Geometry: final body of the model. Coordinates: model frame, mm. A direction names the side the tool comes from. Give positions to 0.01 mm unless a question says otherwise; leave off trailing zeros. Write each loop counter-clockwise with the first axis right and the second up, starting at its lowest first coordinate (ties: lowest second). Pieces come first, ordered by that corner, then holes. Notation, with made-up numbers: M 81,36.5 L 137,36.5 A32 cw 137,62.5 Z; hole C -8,-39 d2. An arc over 180 degrees is marked long. Use a Markdown table: item, result. Add a question column.
1) Line query: line 1 (Y direction, x = -5, z = 27); line 2 (X direction, y = -3.5, z = 4.5); line 3 (X direction, y = -14, z = 16). Output: solid intervals per line, ascending.
2) Section B-B on z = 8. Return the cut outline in (x, y), then the cut area to 3 significant figures.
3) Section D-D on y = 15. Return the cut outline in (x, z).
4) Set-up query: faces 4 (the flat face through (-4, -13.5, 19)), 5 (the flat face through (-1, 0, 23)), 6 (the flat face through (-0.5, 3.15, 34.9)), 7 (the flat face through (-0.5, 3.15, 12.6)). Return all of +Z, -Z, +X, -X, +Y, -Y with unobstructed straight access to the full face (end or side cutting, diameter ignored); none if empty.
5) Pin query (flat end, axial travel): pin 1 (2.5 mm diameter, centred on x = -3, z = 19.5, fed in from -Y); pin 2 (3 mm diameter, centred on y = 16.5, z = 18.5, fed in from +X); pin 3 (2 mm diameter, centred on y = 2, z = 29.5, fed in from -X); pin 4 (3 mm diameter, centred on y = -0.5, z = 6.5, fed in from +X). Return the tip coordinate at first contact, or that it passes through.
6) Section A-A on x = -3.25. Return the cut outline in (y, z), then the cut area to 3 significant figures.
7) Draft query along Z for faces 1 (the cylindrical face through (-0.5, -0.1, 21.5)), 2 (the flat face through (-0.7, 0.1, 0)), 3 (the flat face through (-4, 13.5, 19)). Return one class per face: +Z half, -Z half, draft (parallel to the pull), parting line (faces both ways), or undercut.
8) Section C-C on z = 27.5. Return the cut outline in (x, y), then the cut area to 3 significant figures.
```python
from build123d import *

# Parameters (mm, degrees)
EXTRUDE_THIN1_DEPTH = 50.8
CUT_EXTRUDE1_START  = -8.5
CUT_EXTRUDE1_DEPTH  = 9.5
LPATTERN1_COUNT     = 2
LPATTERN1_PITCH     = 25
FILLET1_R           = 0.25
FILLET2_R           = 1.25
SKETCH5_W           = 12.8
SKETCH5_H           = 35
CUT_EXTRUDE2_DEPTH  = 8.5


with BuildPart() as part:
    # Sketch3 → Extrude-Thin1 (new body)
    with BuildSketch(Plane.XY):
        Polygon((-6.5, 17.5), (-6.5, 13.5), (0, 13.5), (0, -13.5), (-6.5, -13.5), (-6.5, -17.5), (-7.5, -17.5), (-7.5, -12.5), (-1, -12.5), (-1, 12.5), (-7.5, 12.5), (-7.5, 17.5), align=None)
    extrude(amount=EXTRUDE_THIN1_DEPTH)

    # Sketch4 → Cut-Extrude1 (cut)
    with BuildSketch(Plane(origin=(0, 0, 0), x_dir=(0, 0, -1), z_dir=(1, 0, 0)).offset(CUT_EXTRUDE1_START)):
        with BuildLine():
            Line((-6.65, -3.15), (-18.35, -3.15))
            ThreePointArc((-18.35, -3.15), (-21.5, 0), (-18.35, 3.15))
            Line((-18.35, 3.15), (-6.65, 3.15))
            ThreePointArc((-6.65, 3.15), (-3.5, 0), (-6.65, -3.15))
        make_face()
    cut_extrude1 = extrude(amount=CUT_EXTRUDE1_DEPTH, mode=Mode.SUBTRACT)

    # LPattern1: Cut-Extrude1 ×2
    with Locations(*[(0, 0, i * LPATTERN1_PITCH) for i in range(1, LPATTERN1_COUNT)]):
        add(cut_extrude1, mode=Mode.SUBTRACT)

    # Fillet1
    fillet1_edges = [part.edges().sort_by_distance(p)[0] for p in [
        (-6.5, 13.5, 25.4),
        (-6.5, -13.5, 25.4),
        (-1, -12.5, 25.4),
        (-1, 12.5, 25.4),
    ]]
    fillet(fillet1_edges, radius=FILLET1_R)

    # Fillet2
    fillet2_edges = [part.edges().sort_by_distance(p)[0] for p in [
        (0, 13.5, 25.4),
        (0, -13.5, 25.4),
        (-7.5, -12.5, 25.4),
        (-7.5, 12.5, 25.4),
    ]]
    fillet(fillet2_edges, radius=FILLET2_R)

    # Sketch5 → Cut-Extrude2 (cut, through all)
    with BuildSketch(Plane.ZY.offset(7.5)):
        with Locations((44.4, 0)):
            Rectangle(SKETCH5_W, SKETCH5_H)
    extrude(amount=-CUT_EXTRUDE2_DEPTH, mode=Mode.SUBTRACT)


solid = part.part
```
Found:
| question | item | result |
|---|---|---|
| 1 | line 1 | -13.5 to -12.5, 12.5 to 13.5 |
| 1 | line 2 | -1 to 0 |
| 1 | line 3 | -7.5 to -6.5 |
| 2 | outline | M -7.5,-17.5 L -6.5,-17.5 L -6.5,-13.75 A0.25 cw -6.25,-13.5 L -1.25,-13.5 A1.25 ccw 0,-12.25 L 0,-3.15 L -1,-3.15 L -1,-12.25 A0.25 cw -1.25,-12.5 L -6.25,-12.5 A1.25 ccw -7.5,-13.75 Z; M -7.5,13.75 A1.25 ccw -6.25,12.5 L -1.25,12.5 A0.25 cw -1,12.25 L -1,3.15 L 0,3.15 L 0,12.25 A1.25 ccw -1.25,13.5 L -6.25,13.5 A0.25 cw -6.5,13.75 L -6.5,17.5 L -7.5,17.5 Z |
| 2 | area | 40.4 mm² |
| 3 | outline | M -7.5,0 L -6.5,0 L -6.5,38 L -7.5,38 Z |
| 4 | face 4 | +Z, -Z, +X, -Y |
| 4 | face 5 | +Z, -Z, -X |
| 4 | face 6 | +Z, +X, -X |
| 4 | face 7 | +X, -X |
| 5 | pin 1 | y = -13.5 |
| 5 | pin 2 | x = -6.5 |
| 5 | pin 3 | x = -1 |
| 5 | pin 4 | through |
| 6 | outline | M -13.5,0 L -12.5,0 L -12.5,38 L -13.5,38 Z; M 12.5,0 L 13.5,0 L 13.5,38 L 12.5,38 Z |
| 6 | area | 76.0 mm² |
| 7 | face 1 | undercut |
| 7 | face 2 | -Z half |
| 7 | face 3 | draft |
| 8 | outline | M -7.5,-17.5 L -6.5,-17.5 L -6.5,-13.75 A0.25 cw -6.25,-13.5 L -1.25,-13.5 A1.25 ccw 0,-12.25 L 0,12.25 A1.25 ccw -1.25,13.5 L -6.25,13.5 A0.25 cw -6.5,13.75 L -6.5,17.5 L -7.5,17.5 L -7.5,13.75 A1.25 ccw -6.25,12.5 L -1.25,12.5 A0.25 cw -1,12.25 L -1,-12.25 A0.25 cw -1.25,-12.5 L -6.25,-12.5 A1.25 ccw -7.5,-13.75 Z |
| 8 | area | 46.7 mm² |
